Part model, mm, in its own coordinate system. Give positions to 0.01 mm unless a question says otherwise; leave off trailing zeros. Loops run counter-clockwise (first coordinate to the right, second up) from the corner with the lowest first, then second, coordinate; pieces in that order, holes last. Notation, with made-up numbers: (61.5, 68.5) -> (113.5, 68.5) arc R19 cw to (113.5, 95.5) -> close; hole circle Ø8 at (4.25, 55). An arc over 180 degrees is marked (long way). Write item = value, one per line.
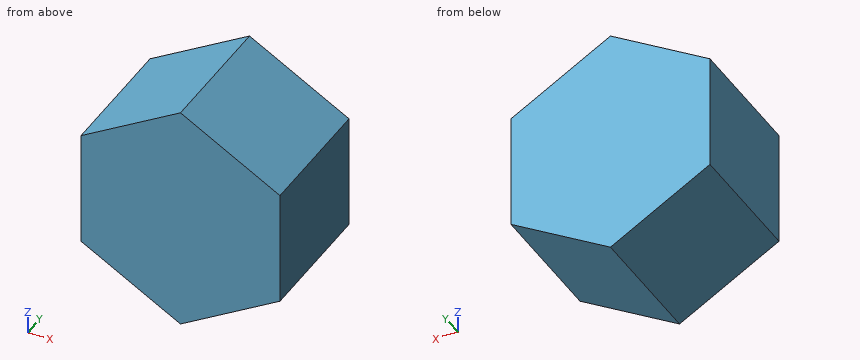
Autodesk Inventor part; units mm, degrees
ref_plane "YZ Plane" through (0, 0, 0) normal (1, 0, 0) x (0, 1, 0)
ref_plane "XZ Plane" through (0, 0, 0) normal (0, 1, 0) x (-1, 0, 0)
ref_plane "XY Plane" through (0, 0, 0) normal (0, 0, 1) x (1, 0, 0)
sketch "Sketch1" plane through (0, 0, 0) normal (0, 1, 0) x (-1, 0, 0)
  line L0 (0, -692.8203) -> (-600, -346.4102)
  line L1 (-600, -346.4102) -> (-600, 346.4102)
  line L2 (-600, 346.4102) -> (0, 692.8203)
  line L3 (0, 692.8203) -> (600, 346.4102)
  line L4 (600, 346.4102) -> (600, -346.4102)
  line L5 (600, -346.4102) -> (0, -692.8203)
  point P0 (0, 0)
  point P1 (0, 0)
  dimension "d0" = 1200
extrude "Extrusion1" add sketch "Sketch1" along normal blind 800
sketch "Sketch2" plane through (600, 0, 346.4102) normal (0.5, 0, 0.866) x (0.866, 0, -0.5)
  line L0 (-692.8203, 0) -> (-692.8203, 800)
  line L1 (-692.8203, 400) -> (0, 400)
  line L2 (0, 0) -> (0, 800)
  point P0 (-346.4102, 0)
  dimension "d3" = 400
sketch "Sketch3" plane through (600, 0, 346.4102) normal (1, 0, 0) x (0, 0, -1)
  line L0 (0, 0) -> (0, 800)
  line L1 (0, 400) -> (692.8203, 400)
  line L2 (692.8203, 0) -> (692.8203, 800)
  point P0 (346.4102, 0)
sketch "Sketch4" plane through (0, 0, -692.8203) normal (0.5, 0, -0.866) x (-0.866, 0, -0.5)
  line L0 (-692.8203, 0) -> (-692.8203, 800)
  line L1 (-692.8203, 400) -> (0, 400)
  line L2 (0, 0) -> (0, 800)
  point P0 (-346.4102, 0)
sketch "Sketch5" plane through (0, 0, 692.8203) normal (-0.5, 0, 0.866) x (0.866, 0, 0.5)
  line L0 (0, 400) -> (-692.8203, 400)
  point P0 (-346.4102, 0)
sketch "Sketch6" plane through (-600, 0, -346.4102) normal (-1, 0, 0) x (0, 0, 1)
  line L0 (692.8203, 400) -> (0, 400)
  point P0 (346.4102, 0)
sketch "Sketch7" plane through (-600, 0, -346.4102) normal (-0.5, 0, -0.866) x (-0.866, 0, 0.5)
  line L0 (0, 400) -> (-692.8203, 400)
  point P0 (-346.4102, 0)
1) Slice it at B-B, the plane x = 159. List the corners of the cut face in (y, z), and give its area (3 significant figures).
Resolved:
outline = (0, -601.02) -> (800, -601.02) -> (800, 601.02) -> (0, 601.02) -> close
area = 962,000 mm²
2) Drop flat-ended pins along their axis: P1, Ø3, axis at x = -302, y = 508.5, coming from the +Z side; P2, Ø1, axis at y = 164.5, z = -422, coming from the +X side; P3, Ø4, axis at x = -64, y = 434, coming from the +Z side; P4, Ø2, axis at x = -195, z = 134, coming from the -Y side. Give the stop position or say it passes through.
Resolved:
P1 = 519.33
P2 = 469.94
P3 = 657.02
P4 = 0
3) Slice it at C-C, the plane z = -536. List the corners of the cut face in (x, y).
Resolved:
outline = (-271.62, 0) -> (271.62, 0) -> (271.62, 800) -> (-271.62, 800) -> close
4) Slice it at A-A, the plane y = 536. List the corners of the cut face in (x, z), and give its area (3 significant figures).
Resolved:
outline = (-600, -346.41) -> (0, -692.82) -> (600, -346.41) -> (600, 346.41) -> (0, 692.82) -> (-600, 346.41) -> close
area = 1,250,000 mm²
5) Drill centre lines: line 1 along X through (y, z) = (147, 522.5); line 2 along Z through (x, y) = (-333.5, 488); line 3 along X through (y, z) = (569, 473.5). Where is each one in solid material? Low to high. Write a range as [from, to].
Resolved:
line_1 = [-295, 295]
line_2 = [-500.27, 500.27]
line_3 = [-379.87, 379.87]
